Source: three-view drawing plus pictorial views. Frame: mm from the lowest corner of the part. Give positions to 0.01 mm unless a question says otherwise; leave off trailing zeros. Write each loop counter-clockwise with the first axis right and the second up, starting at its lowest first coordinate (ties: lowest second). Pieces come first, ordered by that corner, then holes.
Q1. Draft query along Z for the marked faces 1 and 2. Return one class per face: pulls with the +Z half, pulls with the -Z half, needs draft (parallel to the pull), parting line crosses it, or undercut.
Q2. Pin query (flat end, axial travel): pin 1 (3 mm diameter, centred on y = 171.5, z = 11, fed in from +X); pin 2 (4 mm diameter, centred on x = 9.5, y = 156.5, fed in from +Z); pin 3 (1.5 mm diameter, centred on x = 18, y = 117, fed in from +Z). Return the tip coordinate at first contact, or that it passes through.
Q3. Cut plane C-C on y = 143.5. Return the cut outline in (x, z) (3 decimals), plus the area to 3 significant figures.
Q4. Cut plane B-B on x = 11.5. Return the cut outline in (y, z).
Q5. Line query: L1, parallel to Z at x = 12.7, y = 70 (3 decimals); L2, parallel to X at y = 152, z = 16.5; L3, parallel to X at y = 183.5, z = 8.5. Output: solid intervals per line, ascending.
Q6. Cut plane A-A on z = 12.7. Return the cut outline in (x, y) (3 decimals), plus the area to 3 significant figures.
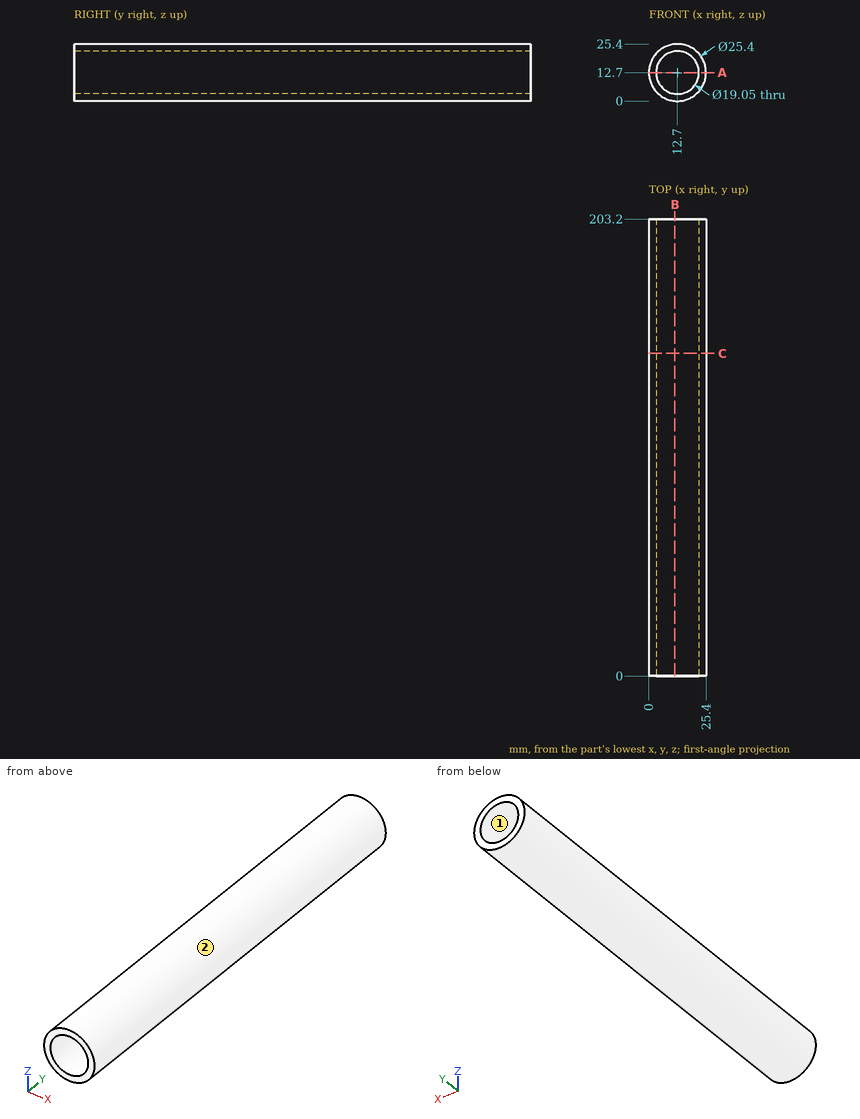
Data:
1. face 1: undercut
1. face 2: parting line crosses it
2. pin 1: stops at x = 25.4
2. pin 2: stops at z = 25.34
2. pin 3: stops at z = 24.56
3. outline: circle Ø25.4 at (12.7, 12.7); hole circle Ø19.05 at (12.7, 12.7)
3. area: 222 mm2
4. outline: (0, 0.06) - (203.2, 0.06) - (203.2, 3.25) - (0, 3.25) - close; (0, 22.15) - (203.2, 22.15) - (203.2, 25.34) - (0, 25.34) - close
5. L1: z = 0 to 3.175, 22.225 to 25.4
5. L2: x = 0.58 to 3.97, 21.43 to 24.82
5. L3: x = 0.71 to 4.15, 21.25 to 24.69
6. outline: (0, 0) - (3.175, 0) - (3.175, 203.2) - (0, 203.2) - close; (22.225, 0) - (25.4, 0) - (25.4, 203.2) - (22.225, 203.2) - close
6. area: 1,290 mm2
